The model under review builds one solid part; all positions refer to its coordinate system, in mm. A direction names the side the tool comes from. Round coordinates to 2 decimals unless told otherwise and drop trailing zeros. Write each loop counter-clockwise with the first axis right and the second up, starting at its lowest first coordinate (ties: lowest second). Pieces come first, ordered by that corner, then holes. Notation, with made-up numbers: (76, 30.25) -> (88, 30.25) arc R21 cw to (88, 63.25) -> close; hole circle Ø1 at (23, 80.25). An arc over 180 degrees is marked (long way). Return JSON: item names as keys, results as strings. Group by question number.
1. Take a section at B-B, the plane x = 77. Write out the cut boundary in (y, z), then the cut area to 3 significant figures.
2. Mouldability with a two-part tool opening along X and no side actions: class faces 5 (the flat face through (7, -63, -27.221)), 6 (the flat face through (101.6, -45, 10)), 7 (the flat face through (0, -45, 10)), 8 (the flat face through (86.936, -44, -1)) as pulls with the +X half, pulls with the -X half, needs draft (parallel to the pull), parting line crosses it, or undercut.
3. Take a section at A-A, the plane z = 3. Write out the cut boundary in (x, y), then the cut area to 3 significant figures.
4. Clearance check with flat-ended pins moving along their axes: P1, Ø5, axis at x = 93, y = -62.5, coming from the -Z side; P2, Ø4, axis at x = 11.5, z = 17.5, coming from the -Y side; P3, Ø15, axis at x = 60, y = -38, coming from the +Z side. State where each tip first meets the part, or that it passes through.
5. Tool access review of faces 1 (the flat face through (94, -63, -27.221)), 2 (the flat face through (50, -38, 21.903)), 3 (the flat face through (50, -23.042, 8)), 4 (the flat face through (6.803, -57.533, -15.473)): name each direction out of +Z, -Z, +X, -X, +Y, -Y from which nothing blocks a thin tool from reaching the whole face with its end or side.
6. Take a section at C-C, the plane z = -6. Write out the cut boundary in (x, y).
7. Take a section at D-D, the plane y = -25.5. Write out the cut boundary in (x, z).
8. For line 1 along X through (y, z) = (-28.5, -17); line 2 along Z through (x, y) = (40.5, -43.5); line 3 along Z through (x, y) = (93.5, -41.5), list the stretches that pass through material, from the lowest coordinate up. Write a range as from..to.
from build123d import *

# Parameters (mm, degrees)
F1_DEPTH = 101.6
F2_W     = 73.136294
F2_H     = 31.528215
F3_DEPTH = 43.25955
F4_R     = 5.08


with BuildPart() as f1:
    # F0 (on Right) → F1 (new body)
    with BuildSketch(Plane.YZ):
        Polygon((-66.300608, 46.098899), (-66.231251, 41.988105), (-66.231251, -27.220687), (-59.701849, -27.220687), (-55.302672, -3.391821), (-31.840406, -3.391821), (-30.374017, -27.403988), (-23.042059, -27.403988), (-23.042059, -3.025223), (-23.042059, 21.903437), (-53.469684, 21.903437), (-59.885152, 46.098899), align=None)
    extrude(amount=F1_DEPTH)

    # F2 (on face) → F3 (cut, through all)
    with BuildSketch(Plane(origin=(0, -23.042059, 0), x_dir=(-1, 0, 0), z_dir=(0, 1, 0))):
        with Locations((-50.367939, -11.639881)):
            Rectangle(F2_W, F2_H)
    extrude(amount=-F3_DEPTH, mode=Mode.SUBTRACT)

    # F4
    f4_edges = [f1.edges().sort_by_distance(p)[0] for p in [
        (50.8, -59.885152, 46.098899),
    ]]
    fillet(f4_edges, radius=F4_R)


solid = f1.part
Output:
{
 "1": {"outline": "(-66.3, 46.1) -> (-66.23, 41.99) -> (-66.23, 4.12) -> (-23.04, 4.12) -> (-23.04, 21.9) -> (-53.47, 21.9) -> (-58.88, 42.32) arc R5.08 ccw to (-63.79, 46.1) -> close", "area": "996 mm^2"},
 "2": {"face 5": "needs draft", "face 6": "pulls with the +X half", "face 7": "pulls with the -X half", "face 8": "undercut"},
 "3": {"outline": "(0, -66.23) -> (13.8, -66.23) -> (13.8, -23.04) -> (0, -23.04) -> close; (86.94, -66.23) -> (101.6, -66.23) -> (101.6, -23.04) -> (86.94, -23.04) -> close", "area": "1,230 mm^2"},
 "4": {"P1": "stops at z = -27.22", "P2": "stops at y = -66.23", "P3": "stops at z = 21.9"},
 "5": {"face 1": "-Z, +X, -X, -Y", "face 2": "+Z, +X, -X, +Y", "face 3": "+Z, -Z, +X, -X, +Y", "face 4": "-Z, +X, -X"},
 "6": {"outline": "(0, -66.23) -> (13.8, -66.23) -> (13.8, -55.78) -> (0, -55.78) -> close; (0, -31.68) -> (13.8, -31.68) -> (13.8, -23.04) -> (0, -23.04) -> close; (86.94, -66.23) -> (101.6, -66.23) -> (101.6, -55.78) -> (86.94, -55.78) -> close; (86.94, -31.68) -> (101.6, -31.68) -> (101.6, -23.04) -> (86.94, -23.04) -> close"},
 "7": {"outline": "(0, -27.4) -> (13.8, -27.4) -> (13.8, 4.12) -> (86.94, 4.12) -> (86.94, -27.4) -> (101.6, -27.4) -> (101.6, 21.9) -> (0, 21.9) -> close"},
 "8": {"line 1": "x = 0..13.8, 86.94..101.6", "line 2": "z = 4.12..21.9", "line 3": "z = -3.39..21.9"}
}
